```python
from build123d import *

# Parameters (mm, degrees)
SKETCH_R            = 2.15
PAD_DEPTH           = 2
POCKET_DEPTH        = 0.001
POCKET_DEPTH_BACK   = 2.001
LINEARPATTERN_COUNT = 2
LINEARPATTERN_PITCH = 61


with BuildPart() as part:
    # Sketch → Pad (new body)
    with BuildSketch(Plane.XY):
        with BuildLine():
            ThreePointArc((0, 5), (-3.043807, 3.966767), (-4.829629, 1.294095))
            Line((-13.111839, -29.615531), (-4.829629, 1.294095))
            ThreePointArc((-13.111839, -29.615531), (-12.248976, -33.953434), (-8.282209, -35.909626))
            Line((180, -35.909626), (-8.282209, -35.909626))
            ThreePointArc((180, -35.909626), (185.815743, -31.385138), (182.860399, -24.635338))
            Line((182.860399, -24.635338), (130, 4.032384))
            ThreePointArc((130, 4.032384), (128.153484, 4.754324), (126.186135, 5))
            Line((0, 5), (126.186135, 5))
        make_face()
        Circle(SKETCH_R, mode=Mode.SUBTRACT)
        with Locations((180, -29.909626)):
            Circle(SKETCH_R, mode=Mode.SUBTRACT)
        with Locations((-8.282209, -30.909626)):
            Circle(SKETCH_R, mode=Mode.SUBTRACT)
        with BuildLine():
            ThreePointArc((173.149083, -27.909626), (174.958635, -26.501845), (174.039088, -24.401663))
            Line((132.953466, -2.119743), (174.039088, -24.401663))
            ThreePointArc((132.953466, -2.119743), (130.976998, -2.159274), (130, -3.877839))
            Line((130, -25.909626), (130, -3.877839))
            ThreePointArc((130, -25.909626), (130.585786, -27.32384), (132, -27.909626))
            Line((132, -27.909626), (173.149083, -27.909626))
        make_face(mode=Mode.SUBTRACT)
    extrude(amount=PAD_DEPTH)

    # Sketch_1 → Pocket (cut, two sides)
    with BuildSketch(Plane.XY) as pocket_sk:
        with BuildLine():
            Line((10.886302, -4.012607), (51.55478, -24.116733))
            ThreePointArc((50.668478, -27.909626), (52.616013, -26.364716), (51.55478, -24.116733))
            Line((50.668478, -27.909626), (10, -27.909626))
            ThreePointArc((8, -25.909626), (8.585786, -27.32384), (10, -27.909626))
            Line((8, -25.909626), (8, -5.805501))
            ThreePointArc((10.886302, -4.012607), (8.944681, -4.106589), (8, -5.805501))
        make_face()
        with BuildLine():
            Line((17.44522, -2.792894), (58.113698, -22.897019))
            ThreePointArc((58.113698, -22.897019), (60.055319, -22.803037), (61, -21.104125))
            Line((61, -21.104125), (61, -1))
            ThreePointArc((61, -1), (60.414214, 0.414214), (59, 1))
            Line((59, 1), (18.331522, 1))
            ThreePointArc((18.331522, 1), (16.383987, -0.544911), (17.44522, -2.792894))
        make_face()
    pocket = extrude(amount=-POCKET_DEPTH, mode=Mode.SUBTRACT) + extrude(pocket_sk.sketch, amount=POCKET_DEPTH_BACK, mode=Mode.SUBTRACT)

    # LinearPattern: Pocket ×2
    with Locations(*[(i * LINEARPATTERN_PITCH, 0, 0) for i in range(1, LINEARPATTERN_COUNT)]):
        add(pocket, mode=Mode.SUBTRACT)


solid = part.part
```
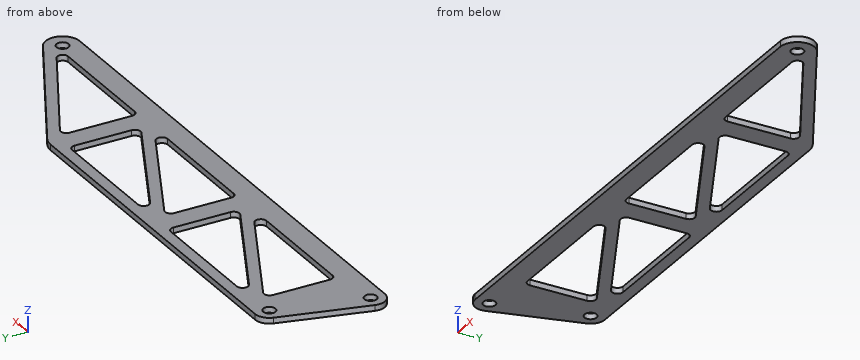
The listing builds one solid part. Answer for the finished solid, in the listing's coordinates (mm). Round coordinates to 2 decimals unless told otherwise and drop trailing zeros. Order: outer loops, then holes, each group sorted by start corner. A loop starts at its lowest first (then second) coordinate and runs counter-clockwise, first axis right, second up. Notation, with made-up numbers: (-11, -31) -> (41, -31) arc R14 ccw to (41, -12) -> close; hole circle Ø5 at (17, 88). An arc over 180 degrees is marked (long way). Answer as CSV lines item,"result". Start each with the question number.
(1) The part is cut by section C-C (z = 1.15). Count the separate pieces of the cut face and the enclosed holes in it, then the cut area to 3 significant figures.
(2) The part is cut by section A-A (y = -16.5). Determine the outline of the cut face in (x, z), then the cut area to 3 significant figures.
(3) Flat-ended cylindrical pins translate along their axes: pin 1 Ø4 at (x, y) = (0, 0) entering from -Z; pin 2 Ø1 at (y, z) = (-11.5, 0.5) entering from -X; pin 3 Ø0.6 at (y, z) = (-15, 0.5) entering from +X; pin 4 Ø0.6 at (x, z) = (160.5, 1.5) entering from +Y. Find the tip coordinate at first contact, or state that the pin passes through.
(4) The part is cut by section B-B (x = 160.5). Determine the outline of the cut face in (y, z).
(5) Find the intervals of material crossed by probe 1 along X at (y, z) = (-24, 0.2); probe 2 along Y at (x, z) = (89, 1.5); probe 3 along X at (y, z) = (-31, 0.3), in increasing order. Write a range as from..to.
Evaluation:
1,separate pieces,"1"
1,enclosed holes,"8"
1,area,"3,800 mm²"
2,outline,"(-9.6, 0) -> (8, 0) -> (8, 2) -> (-9.6, 2) -> close; (36.15, 0) -> (45.17, 0) -> (45.17, 2) -> (36.15, 2) -> close; (61, 0) -> (69, 0) -> (69, 2) -> (61, 2) -> close; (97.15, 0) -> (106.17, 0) -> (106.17, 2) -> (97.15, 2) -> close; (122, 0) -> (130, 0) -> (130, 2) -> (122, 2) -> close; (159.47, 0) -> (167.86, 0) -> (167.86, 2) -> (159.47, 2) -> close"
2,area,"120 mm²"
3,pin 1,"through"
3,pin 2,"x = -8.39"
3,pin 3,"x = 165.65"
3,pin 4,"y = -12.35"
4,outline,"(-35.91, 0) -> (-27.91, 0) -> (-27.91, 2) -> (-35.91, 2) -> close; (-17.06, 0) -> (-12.51, 0) -> (-12.51, 2) -> (-17.06, 2) -> close"
5,probe 1,"-11.61..8, 51.32..69, 112.32..130, 173.3..181.69"
5,probe 2,"-35.91..-27.91, -12.47..-8.01, 1..5"
5,probe 3,"-13.28..-10.43, -6.13..178.15, 181.85..185.9"
